Design review of the part shown in the three views and the two pictorial views. Dimensions are in mm from the part's minimum x, y and z. A direction names the side the tool comes from. Round coordinates to 2 decimals unless told otherwise and drop trailing zeros. Order: outer loops, then holes, each group sorted by start corner. A loop starts at its lowest first (then second) coordinate and runs counter-clockwise, first axis right, second up. Notation, with made-up numbers: M 34,55.5 L 76,55.5 A34 ccw 76,87.5 Z; hole C -1.5,1 d7. An arc over 180 degrees is marked long. Use a Markdown table: item, result. Add a question column.
(1) For pin 1 (3 mm diameter, centred on x = 676, z = 184.5, fed in from +Y) (1 decimal); pin 2 (3 mm diameter, centred on x = 1199, z = 136.5, fed in from -Y); pin 3 (2 mm diameter, centred on x = 231, y = 1106.5, fed in from -Z) (1 decimal), all flat-tipped, find the tip position at first contact; note any pin that passes through.
(2) Take a section at A-A (z = 360). Write out the cut boundary in (x, y) (1 decimal), then the cut area to 3 significant figures.
(3) Machinability: for the marked faces 1 and 2, which of the approach directions +Z, -Z, +X, -X, +Y, -Y give a long, thin tool a straight path to every point of the face, cutting with its end or side? Answer none if there is none.
(4) To check wall thickness, follow probe 1 along Y at (x, z) = (401, 213.5) (1 decimal); probe 2 along Y at (x, z) = (522.5, 348) (1 decimal); probe 3 along X at (y, z) = (790.5, 243.5) (1 decimal). State the ranges of each line that lie inside material, in increasing order. Write a range as from..to.
(5) Take a section at B-B (z = 53.5). Write out the cut boundary in (x, y).
(6) Take a section at C-C (z = 139). Write out the cut boundary in (x, y).
(7) The part is to be moulded in two halves that separate along X. For the marked faces 3, 4, 5 and 6, say which applies: released by +X, released by -X, zero draft, split by the parting line, or undercut.
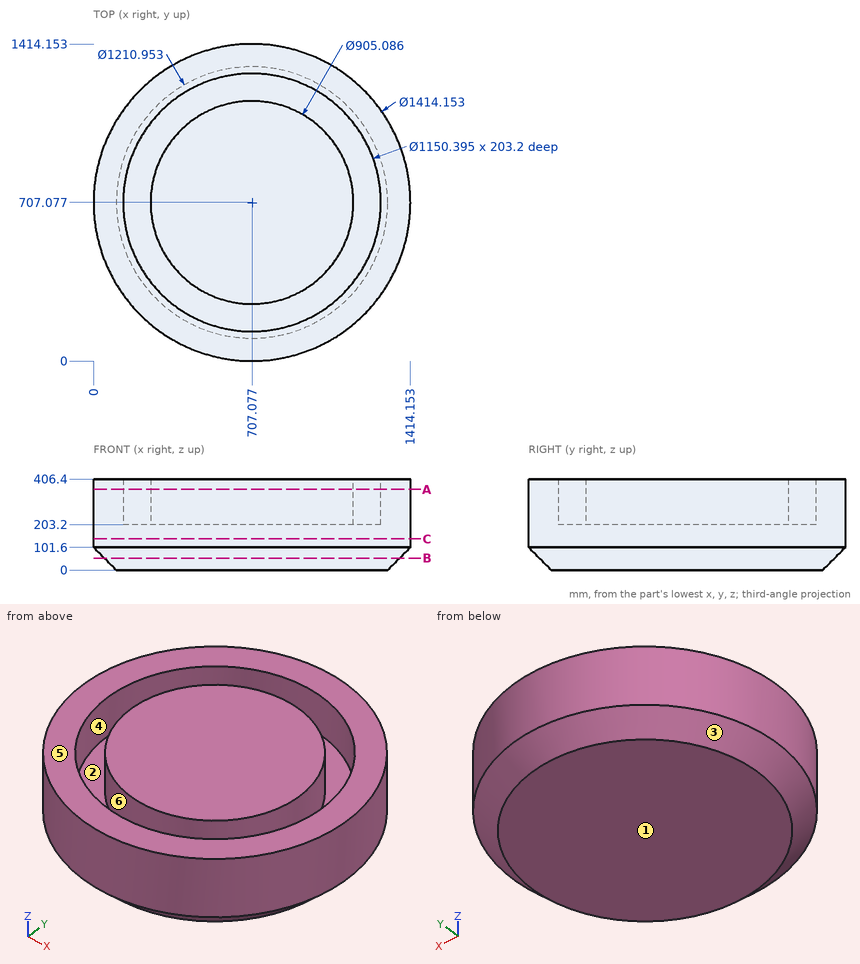
Verdict:
| question | item | result |
|---|---|---|
| 1 | pin 1 | stops at y = 1413.5 |
| 1 | pin 2 | stops at y = 197.72 |
| 1 | pin 3 | stops at z = 15 |
| 2 | outline | C 707.1,707.1 d1414.2; C 707.1,707.1 d905.1; hole C 707.1,707.1 d1150.4 |
| 2 | area | 1,170,000 mm^2 |
| 3 | face 1 | -Z, +X, -X, +Y, -Y |
| 3 | face 2 | +Z |
| 4 | probe 1 | y = 69.7..220.1, 373.7..1040.4, 1194.1..1344.5 |
| 4 | probe 2 | y = 24.5..162.3, 293.9..1120.3, 1251.9..1389.6 |
| 4 | probe 3 | x = 4.9..138, 262.3..1151.9, 1276.2..1409.2 |
| 5 | outline | C 707.08,707.08 d1317.95 |
| 6 | outline | C 707.08,707.08 d1414.15 |
| 7 | face 3 | split by the parting line |
| 7 | face 4 | undercut |
| 7 | face 5 | zero draft |
| 7 | face 6 | undercut |
